Autodesk Inventor part; units mm, degrees
ref_plane "XZ Plane" through (0, 0, 0) normal (0, 1, 0) x (-1, 0, 0)
ref_plane "XY Plane" through (0, 0, 0) normal (0, 0, 1) x (1, 0, 0)
sketch "Sketch1" plane through (0, 0, 0) normal (1, 0, 0) x (0, 1, 0)
  line L0 (0, 4.9645) -> (36.2523, 21.8692)
  line L1 (36.2523, 21.8692) -> (47, 9.0606)
  line L2 (45.8, 1.6) -> (45.8, 8.6239)
  line L3 (45.8, 8.6239) -> (35.9249, 20.3925)
  line L4 (35.9249, 20.3925) -> (1.2, 4.2)
  line L5 (0, 4.9645) -> (0, 0)
  line L6 (47, 9.0606) -> (47, 0)
  line L7 (0, 0) -> (9.3, 0)
  line L8 (9.3, 0) -> (9.3, 1.6)
  line L9 (9.3, 1.6) -> (4.8, 1.6)
  line L10 (1.2, 4.2) -> (1.2, 1.6)
  line L11 (45.8, 1.6) -> (42.3, 1.6)
  line L12 (37.8, 1.6) -> (37.8, 0)
  line L13 (37.8, 0) -> (47, 0)
  line L14 (4.8, 1.6) -> (4.8, 0) construction
  line L15 (42.3, 1.6) -> (42.3, 0) construction
  line L16 (42.3, 1.6) -> (37.8, 1.6)
  line L17 (4.8, 1.6) -> (1.2, 1.6)
  dimension "d1" = 1.2
  dimension "d3" = 1.2
  dimension "d4" = 1.2
  dimension "d25" = 40
  dimension "d26" = 25
  dimension "d27" = 1.6
  dimension "d28" = 1.2
  dimension "d29" = 37.5
  dimension "d37" = 105
  dimension "d38" = 4.5
  dimension "d39" = 2.6
  dimension "d42" = 3.5
  dimension "d43" = 3.6
extrude "Extrusion1" add sketch "Sketch1" along normal mid plane 46
sketch "Sketch3" plane through (23, 35.9249, 20.3925) normal (0, 0.4226, -0.9063) x (-1, 0, 0)
  circle A0 centre (3.405, -5.0219) radius 1.05
  circle A1 centre (37.695, -5.0219) radius 1.05
  circle A2 centre (37.695, -27.9329) radius 1.05
  circle A3 centre (3.405, -27.9329) radius 1.05
  line L0 (0, -39.4135) -> (0, 0) construction
  line L1 (46, 0) -> (46, -39.4135) construction
  circle A4 centre (3.405, -5.0219) radius 1.85
  circle A5 centre (37.695, -5.0219) radius 1.85
  circle A6 centre (37.695, -27.9329) radius 1.85
  circle A7 centre (3.405, -27.9329) radius 1.85
  line L2 (11.205, -4.9754) -> (34.795, -4.9754)
  line L3 (34.795, -4.9754) -> (34.795, -28.7754)
  line L4 (34.795, -28.7754) -> (11.205, -28.7754)
  line L5 (11.205, -28.7754) -> (11.205, -4.9754)
  line L6 (23, -4.9754) -> (23, -28.7754) construction
  line L7 (11.205, -16.8754) -> (0, -16.8754) construction
  line L8 (34.795, -16.8754) -> (46, -16.8754) construction
  point P0 (23, -41.1773)
  dimension "d13" = 34.29
  dimension "d14" = 22.911
  dimension "d15" = 2.1
  dimension "d16" = 0.8
  dimension "d17" = 7.8
  dimension "d18" = 2.9
  dimension "d19" = 23.8
  dimension "d44" = 0.0465
extrude "Extrusion2" add sketch "Sketch3" along normal blind 1.7 contours A4 | A5 | A6 | A7
extrude "Extrusion3" cut sketch "Sketch3" against normal up to surface (1.2 mm away) contours L2 L3 L4 L5
sketch "Sketch5" plane through (-23, 0, 0) normal (0, 0, -1) x (-1, 0, 0)
  arc A0 (-4, 3) -> (-4, 6.6) centre (-4, 4.8) ccw
  arc A1 (-42, 6.6) -> (-42, 3) centre (-42, 4.8) ccw
  arc A2 (-42, 44.1) -> (-42, 40.5) centre (-42, 42.3) ccw
  arc A3 (-4, 40.5) -> (-4, 44.1) centre (-4, 42.3) ccw
  line L0 (0, 9.3) -> (0, 0) construction
  line L1 (-46, 9.3) -> (0, 9.3) construction
  line L2 (-46, 0) -> (-46, 9.3) construction
  line L3 (-46, 0) -> (0, 0) construction
  line L4 (0, 47) -> (0, 37.8) construction
  line L5 (-46, 47) -> (0, 47) construction
  line L6 (-46, 37.8) -> (-46, 47) construction
  line L7 (-46, 37.8) -> (0, 37.8) construction
  line L8 (-23, -9.4) -> (-23, 56.4)
  arc A4 (-8, 6.6) -> (-8, 3) centre (-8, 4.8) ccw construction
  line L9 (-4, 6.6) -> (-8, 6.6)
  line L10 (-4, 3) -> (-8, 3)
  arc A5 (-38, 3) -> (-38, 6.6) centre (-38, 4.8) ccw construction
  arc A6 (-38, 40.5) -> (-38, 44.1) centre (-38, 42.3) ccw construction
  arc A7 (-8, 44.1) -> (-8, 40.5) centre (-8, 42.3) ccw construction
  line L11 (-38, 3) -> (-42, 3)
  line L12 (-38, 6.6) -> (-42, 6.6)
  line L13 (-38, 40.5) -> (-42, 40.5)
  line L14 (-42, 44.1) -> (-38, 44.1)
  line L15 (-4, 44.1) -> (-8, 44.1)
  line L16 (-8, 40.5) -> (-4, 40.5)
  arc A8 (-8, 6.6) -> (-8, 3) centre (-10.7659, 4.8) ccw
  arc A9 (-38, 3) -> (-38, 6.6) centre (-35.2341, 4.8) ccw
  arc A10 (-8, 44.1) -> (-8, 40.5) centre (-10.7659, 42.3) ccw
  arc A11 (-38, 40.5) -> (-38, 44.1) centre (-35.2341, 42.3) ccw
  point P0 (-23, 0)
  point P1 (-23, 4.8)
  dimension "d30" = 37.5
  dimension "d31" = 38
  dimension "d32" = 3.6
  dimension "d33" = 4
  dimension "d34" = 6.6
extrude "Extrusion4" cut sketch "Sketch5" against normal up to next
ref_plane "Work Plane1" through (18.75, 0, 0) normal (1, 0, 0) x (0, 1, 0)
ref_plane "Work Plane2" through (-18.75, 0, 0) normal (1, 0, 0) x (0, 1, 0)
ref_plane "Work Plane3" through (15, 42.3, 1.6) normal (0, -1, 0) x (1, 0, 0)
properties part number "DisplayMount"
Can you work these out from the model? Positions are in its coordinate system, mm. A direction names the side the tool comes from. Round coordinates to 2 decimals unless told otherwise and drop trailing zeros. Loops run counter-clockwise (first coordinate to the right, second up) from the corner with the lowest first, then second, coordinate; pieces in that order, holes last. Notation, with made-up numbers: M -12.5,51.25 L 16.5,51.25 A9 cw 16.5,68.25 Z; hole C 36.25,37 d5. An arc over 180 degrees is marked long. Answer in a Markdown table with one row per item.
1. If we section it at D-D, the plane y = 42.3: Please give me the cut outline in (x, z) (3 decimals), plus the area to 3 significant figures.
Established:
| item | result |
|---|---|
| outline | M -23,0 L -20.8,0 L -20.8,1.6 L -23,1.6 Z; M -23,12.795 L 23,12.795 L 23,14.662 L -23,14.662 Z; M -8.934,0 L 8.934,0 L 8.934,1.6 L -8.934,1.6 Z; M 20.8,0 L 23,0 L 23,1.6 L 20.8,1.6 Z |
| area | 122 mm² |
2. I'm going to push flat-ended pins straight in: pin 1 Ø10 at (x, y) = (1, 25) entering from +Z; pin 2 Ø8 at (x, z) = (-7.5, 19) entering from -Y; pin 3 Ø9 at (x, y) = (9.5, 42.5) entering from +Z; pin 4 Ø6 at (x, y) = (-15, 11.5) entering from +Z. Where does each tip first touch, or does it pass through?
Established:
| item | result |
|---|---|
| pin 1 | through |
| pin 2 | y = 30.91 |
| pin 3 | z = 19.79 |
| pin 4 | z = 11.73 |
3. Please list where these lines run through material, in increasing order: line 1 (X direction, y = 4.8, z = 0.55); line 2 (Y direction, x = -11.5, z = 1.5); line 3 (Y direction, x = 14.5, z = 1.25). Write a range as from..to.
Established:
| item | result |
|---|---|
| line 1 | -23..-20.8, -8.93..8.93, 20.8..23 |
| line 2 | 0..1.58, 8.02..9.3, 37.8..39.08, 45.52..47 |
| line 3 | 0..2.4, 7.2..9.3, 37.8..39.9, 44.7..47 |
4. If we section it at B-B, the plane z = 3.5: Please give me the cut outline in (x, y), plus the area to 3 significant figures.
Established:
| item | result |
|---|---|
| outline | M -23,0 L 23,0 L 23,1.2 L -23,1.2 Z; M -23,45.8 L 23,45.8 L 23,47 L -23,47 Z |
| area | 110 mm² |
5. Thinking about a two-plate mould opening in Y: for faces 1 (the face through (17, 6.6, 1)), 2 (the face through (0, 5, 0)), 3 (the face through (0, 1.2, 3)), 4 (the face through (-0.322, 41.551, 15.555)), which applies, pulls with the +Y half, pulls with the -Y half, needs draft (parallel to the pull), parting line crosses it, or undercut?
Established:
| item | result |
|---|---|
| face 1 | undercut |
| face 2 | needs draft |
| face 3 | undercut |
| face 4 | pulls with the +Y half |
6. On a 3-axis mill with a long thin cutter (end or side, diameter ignored), from which of +Z, -Z, +X, -X, +Y, -Y can I reach the whole of each face in a straight line? I mean faces 5 (the face through (0, 5, 1.6)), 6 (the face through (19.58, 10.622, 8.594)), 7 (the face through (-20.8, 4.8, 0.8)), 8 (the face through (0, 9.3, 1)). Say none if no direction works.
Established:
| item | result |
|---|---|
| face 5 | +X, -X |
| face 6 | none |
| face 7 | -Z |
| face 8 | -Z, +X, -X |
7. If we section it at C-C, the plane x = -1.5: Please give me the cut outline in (y, z).
Established:
| item | result |
|---|---|
| outline | M 0,0 L 9.3,0 L 9.3,1.6 L 1.2,1.6 L 1.2,4.2 L 9.85,8.23 L 9.34,9.32 L 0,4.96 Z; M 30.91,19.38 L 31.42,18.29 L 35.92,20.39 L 45.8,8.62 L 45.8,1.6 L 37.8,1.6 L 37.8,0 L 47,0 L 47,9.06 L 36.25,21.87 Z |
8. If we section it at A-A, the plane x = 17: Please give me the cut outline in (y, z), plus the area to 3 significant figures.
Established:
| item | result |
|---|---|
| outline | M 0,0 L 3,0 L 3,1.6 L 1.2,1.6 L 1.2,4.2 L 35.92,20.39 L 45.8,8.62 L 45.8,1.6 L 44.1,1.6 L 44.1,0 L 47,0 L 47,9.06 L 36.25,21.87 L 0,4.96 Z; M 6.6,0 L 9.3,0 L 9.3,1.6 L 6.6,1.6 Z; M 37.8,0 L 40.5,0 L 40.5,1.6 L 37.8,1.6 Z |
| area | 96.6 mm² |
